Read the model definition and answer for the solid it produces. Units are mm, in the model's axes. Coordinates: 2 decimals unless noted, no trailing zeros. Write each loop counter-clockwise with the first axis right and the second up, starting at its lowest first coordinate (ties: lowest second). Pieces come first, ordered by that corner, then holes. Notation, with made-up numbers: (29, -1.75) - (66, -1.75) arc R21 cw to (66, 10.25) - close; hole circle Ø8 at (27.5, -25). An arc over 180 degrees is marked (long way). Return JSON: item names as keys, results as strings.
```python
from build123d import *

# Parameters (mm, degrees)
SKETCH1_W           = 110
SKETCH1_H           = 140
SKETCH1_R           = 2
BOSS_EXTRUDE1_DEPTH = 3.175
SKETCH2_R           = 2.25
BOSS_EXTRUDE2_DEPTH = 3.175
SKETCH3_R           = 45
SKETCH3_R_2         = 2
SKETCH3_R_3         = 13
SKETCH3_R_4         = 1.4732
BOSS_EXTRUDE3_DEPTH = 3.175
BOSS_EXTRUDE5_DEPTH = 3.175
FILLET1_R           = 6
SKETCH6_R           = 2
SKETCH6_R_2         = 13
CUT_EXTRUDE1_DEPTH  = 10


with BuildPart() as part:
    # Sketch1 → Boss-Extrude1 (new body)
    with BuildSketch(Plane.XY):
        Rectangle(SKETCH1_W, SKETCH1_H)
        with Locations((-47.5, 40)):
            Circle(SKETCH1_R, mode=Mode.SUBTRACT)
        with Locations((47.5, 40)):
            Circle(SKETCH1_R, mode=Mode.SUBTRACT)
        with Locations((-47.5, 60)):
            Circle(SKETCH1_R, mode=Mode.SUBTRACT)
        with Locations((47.5, 60)):
            Circle(SKETCH1_R, mode=Mode.SUBTRACT)
    extrude(amount=BOSS_EXTRUDE1_DEPTH)

    # Sketch2 → Boss-Extrude2 (add)
    with BuildSketch(Plane.XY):
        Polygon((-26.715730122, -70), (-55, -41.715730122), (-115, -101.715728753), (-115, -183), (-75, -183), (-75, -118.28427098), align=None)
        with Locations((-95, -165.5)):
            Circle(SKETCH2_R, mode=Mode.SUBTRACT)
        with Locations((-95, -130.5)):
            Circle(SKETCH2_R, mode=Mode.SUBTRACT)
    boss_extrude2 = extrude(amount=BOSS_EXTRUDE2_DEPTH)

    # Mirror1: Boss-Extrude2 across plane
    add(boss_extrude2.mirror(Plane(origin=(0, 0, 0), x_dir=(0, 0, 1), z_dir=(1, 0, 0))))

    # Sketch3 → Boss-Extrude3 (add)
    # profile 1 of 2: a face of its own
    with BuildSketch(Plane.XY.offset(3.175)):
        with Locations((-50, -18)):
            Circle(SKETCH3_R)
        with Locations((-67.5, -18)):
            Circle(SKETCH3_R_2, mode=Mode.SUBTRACT)
        with Locations((-50, -18)):
            Circle(SKETCH3_R_3, mode=Mode.SUBTRACT)
        with Locations((-56.511806663, 18.930290738)):
            Circle(SKETCH3_R_4, mode=Mode.SUBTRACT)
        with Locations((-85.238473279, -5.174244625)):
            Circle(SKETCH3_R_4, mode=Mode.SUBTRACT)
    # profile 2 of 2: a face of its own
    with BuildSketch(Plane.XY.offset(3.175)):
        with Locations((50, -18)):
            Circle(SKETCH3_R)
        with Locations((67.5, -18)):
            Circle(SKETCH3_R_2, mode=Mode.SUBTRACT)
        with Locations((50, -18)):
            Circle(SKETCH3_R_3, mode=Mode.SUBTRACT)
        with Locations((56.511806663, 18.930290738)):
            Circle(SKETCH3_R_4, mode=Mode.SUBTRACT)
        with Locations((85.238473279, -5.174244625)):
            Circle(SKETCH3_R_4, mode=Mode.SUBTRACT)
    extrude(amount=-BOSS_EXTRUDE3_DEPTH)

    # Sketch4 → Boss-Extrude5 (add)
    with BuildSketch(Plane.XY.offset(3.175)):
        with BuildLine():
            Line((-60, -101.715728753), (-60, -40))
            Line((-60, -40), (-89.255572853, -40))
            ThreePointArc((-89.255572853, -40), (-94.594805712, -11.97477772), (-82.00977873, 13.628690546))
            Line((-82.00977873, 13.628690546), (-135, -40))
            Line((-135, -40), (-135, -110))
            Line((-135, -110), (-115, -183))
            Line((-115, -183), (-115, -101.715728753))
            Line((-115, -101.715728753), (-60, -101.715728753))
        make_face()
        with BuildLine():
            Line((-127.5, -102.95), (-122.5, -102.95))
            ThreePointArc((-122.5, -102.95), (-120.45, -105), (-122.5, -107.05))
            Line((-122.5, -107.05), (-127.5, -107.05))
            ThreePointArc((-127.5, -107.05), (-129.55, -105), (-127.5, -102.95))
        make_face(mode=Mode.SUBTRACT)
        with BuildLine():
            ThreePointArc((-122.5, -42.95), (-120.45, -45), (-122.5, -47.05))
            Line((-122.5, -47.05), (-127.5, -47.05))
            ThreePointArc((-127.5, -47.05), (-129.55, -45), (-127.5, -42.95))
            Line((-127.5, -42.95), (-122.5, -42.95))
        make_face(mode=Mode.SUBTRACT)
    boss_extrude5 = extrude(amount=-BOSS_EXTRUDE5_DEPTH)

    # Mirror2: Boss-Extrude5 across plane
    add(boss_extrude5.mirror(Plane(origin=(0, 0, 0), x_dir=(0, 0, 1), z_dir=(1, 0, 0))))

    # Fillet1
    fillet1_edges = [part.edges().sort_by_distance(p)[0] for p in [
        (-55, 26.72135955, 1.5875),
        (55, 26.72135955, 1.5875),
    ]]
    fillet(fillet1_edges, radius=FILLET1_R)

    # Sketch6 → Cut-Extrude1 (cut)
    with BuildSketch(Plane.XY.offset(3.175)):
        with Locations((32.5, -18)):
            Circle(SKETCH6_R)
        with Locations((50, -0.5)):
            Circle(SKETCH6_R)
        with Locations((67.5, -18)):
            Circle(SKETCH6_R)
        with Locations((50, -18)):
            Circle(SKETCH6_R_2)
        with Locations((50, -35.5)):
            Circle(SKETCH6_R)
        with Locations((-50, -18)):
            Circle(SKETCH6_R_2)
        with Locations((-67.5, -18)):
            Circle(SKETCH6_R)
        with Locations((-50, -35.5)):
            Circle(SKETCH6_R)
        with Locations((-32.5, -18)):
            Circle(SKETCH6_R)
        with Locations((-50, -0.5)):
            Circle(SKETCH6_R)
    extrude(amount=-CUT_EXTRUDE1_DEPTH, mode=Mode.SUBTRACT)


solid = part.part
```
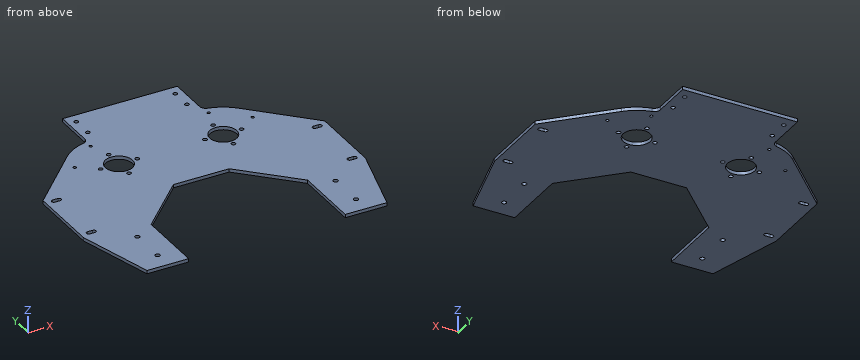
(1) A cutting plane is placed at D-D (x = -101.5). Determine the outline of the cut face in (y, z) (3 decimals).
Answer:
{"outline": "(-183, 0) - (-6.096, 0) - (-6.096, 3.175) - (-183, 3.175) - close"}
(2) A cutting plane is placed at A-A (y = -125). Determine the outline of the cut face in (x, z) (3 decimals), and give its area (3 significant figures).
Answer:
{"outline": "(-130.89, 0) - (-75, 0) - (-75, 3.175) - (-130.89, 3.175) - close; (75, 0) - (130.89, 0) - (130.89, 3.175) - (75, 3.175) - close", "area": "355 mm²"}
(3) A cutting plane is placed at B-B (y = 51). Determine the outline of the cut face in (x, z) (3 decimals), and give its area (3 significant figures).
Answer:
{"outline": "(-55, 0) - (55, 0) - (55, 3.175) - (-55, 3.175) - close", "area": "349 mm²"}
(4) Straight lines are drawn through the part: line 1 (Y direction, x = -47.5, z = 1.8); line 2 (Y direction, x = -46, z = 1); line 3 (X direction, y = -7, z = 0.6). For each, find the intervals that lie inside material, in ascending order. Write a range as from..to.
Answer:
{"line 1": "-90.78..-30.76, -5.24..38, 42..58, 62..70", "line 2": "-89.28..-30.37, -5.63..38.68, 41.32..58.68, 61.32..70", "line 3": "-102.39..-56.93, -43.07..43.07, 56.93..102.39"}
(5) A flat-ended cylindrical pin translates along its axis: P1, Ø1, axis at x = -86, z = 2.5, coming from the +Y side. Find the tip coordinate at first contact, or state that the pin passes through.
Answer:
{"P1": "y = 10.1"}
(6) A cutting plane is placed at C-C (z = 1.6). State how many separate pieces and enclosed holes the cut face has, and give its area (3 significant figures).
Answer:
{"separate pieces": "1", "enclosed holes": "26", "area": "39,400 mm²"}
